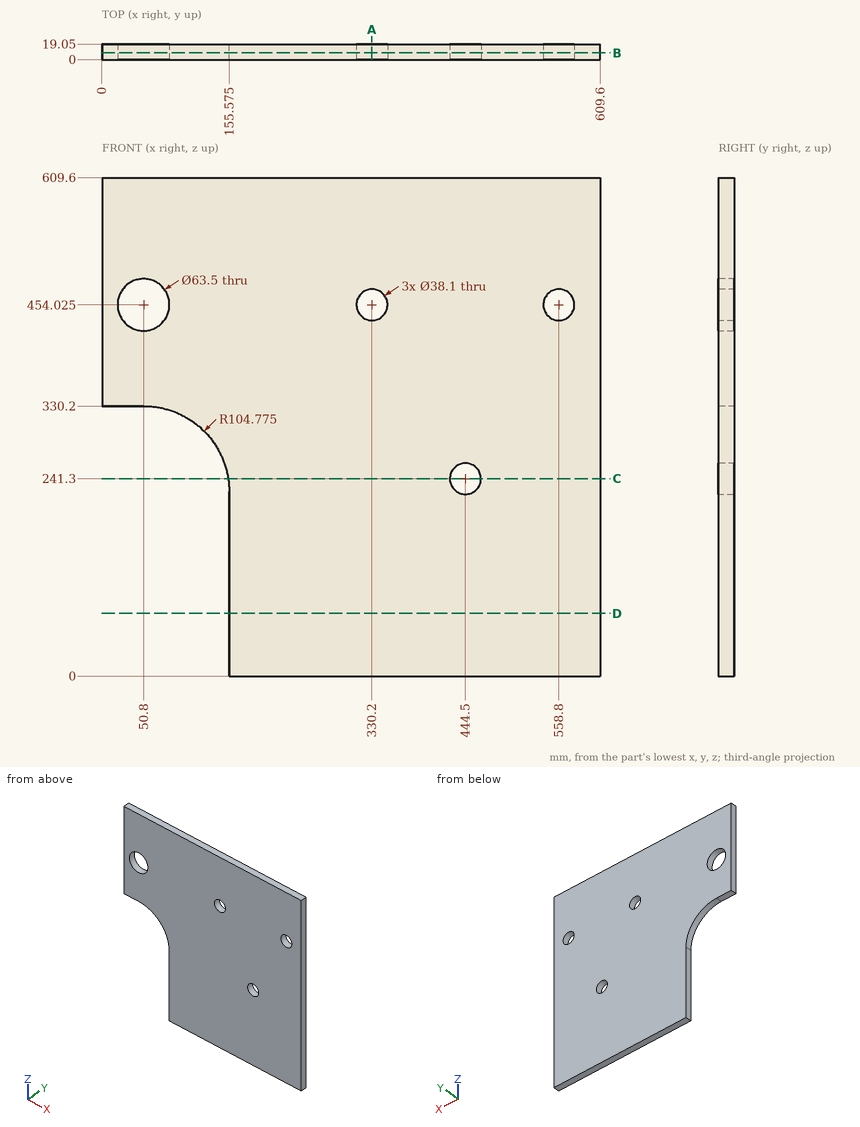
Study the drawing (mm; zero at the part's minimum x, y, z) and answer. Coordinates: 2 decimals unless noted, no trailing zeros. Loops run counter-clockwise (first coordinate to the right, second up) from the corner with the lowest first, then second, coordinate; pieces in that order, holes last. Notation, with made-up numbers: (6, 16) -> (37, 16) arc R26 ccw to (37, 43) -> close; hole circle Ø10 at (58, -36). An arc over 180 degrees is marked (long way). Write each question's results on one line, items separated by ' | '. Start each with the question number.
1) Consider line 1 along X through (y, z) = (4.75, 452); line 2 along X through (y, z) = (4.5, 241.3); line 3 along X through (y, z) = (14.25, 190) (3 decimals). Determine where each line is inside the solid, lowest interval first.
2) Find section B-B on y = 8.25. Determine the outline of the cut face in (x, z) (3 decimals).
3) Find section A-A on x = 330.2. Determine the outline of the cut face in (y, z) (3 decimals).
4) Find section C-C on z = 241.3. Determine the outline of the cut face in (x, y), then the cut area to 3 significant figures.
5) Find section D-D on z = 76.5. Determine the outline of the cut face in (x, y) (3 decimals), then the cut area to 3 significant figures.
Response values:
1) line 1: x = 0 to 19.11, 82.49 to 311.26, 349.14 to 539.86, 577.74 to 609.6 | line 2: x = 154.37 to 425.45, 463.55 to 609.6 | line 3: x = 155.575 to 609.6
2) outline: (0, 330.2) -> (50.8, 330.2) arc R104.775 cw to (155.575, 225.425) -> (155.575, 0) -> (609.6, 0) -> (609.6, 609.6) -> (0, 609.6) -> close; hole circle Ø63.5 at (50.8, 454.025); hole circle Ø38.1 at (330.2, 454.025); hole circle Ø38.1 at (444.5, 241.3); hole circle Ø38.1 at (558.8, 454.025)
3) outline: (0, 0) -> (19.05, 0) -> (19.05, 434.975) -> (0, 434.975) -> close; (0, 473.075) -> (19.05, 473.075) -> (19.05, 609.6) -> (0, 609.6) -> close
4) outline: (154.37, 0) -> (425.45, 0) -> (425.45, 19.05) -> (154.37, 19.05) -> close; (463.55, 0) -> (609.6, 0) -> (609.6, 19.05) -> (463.55, 19.05) -> close | area: 7,950 mm^2
5) outline: (155.575, 0) -> (609.6, 0) -> (609.6, 19.05) -> (155.575, 19.05) -> close | area: 8,650 mm^2
